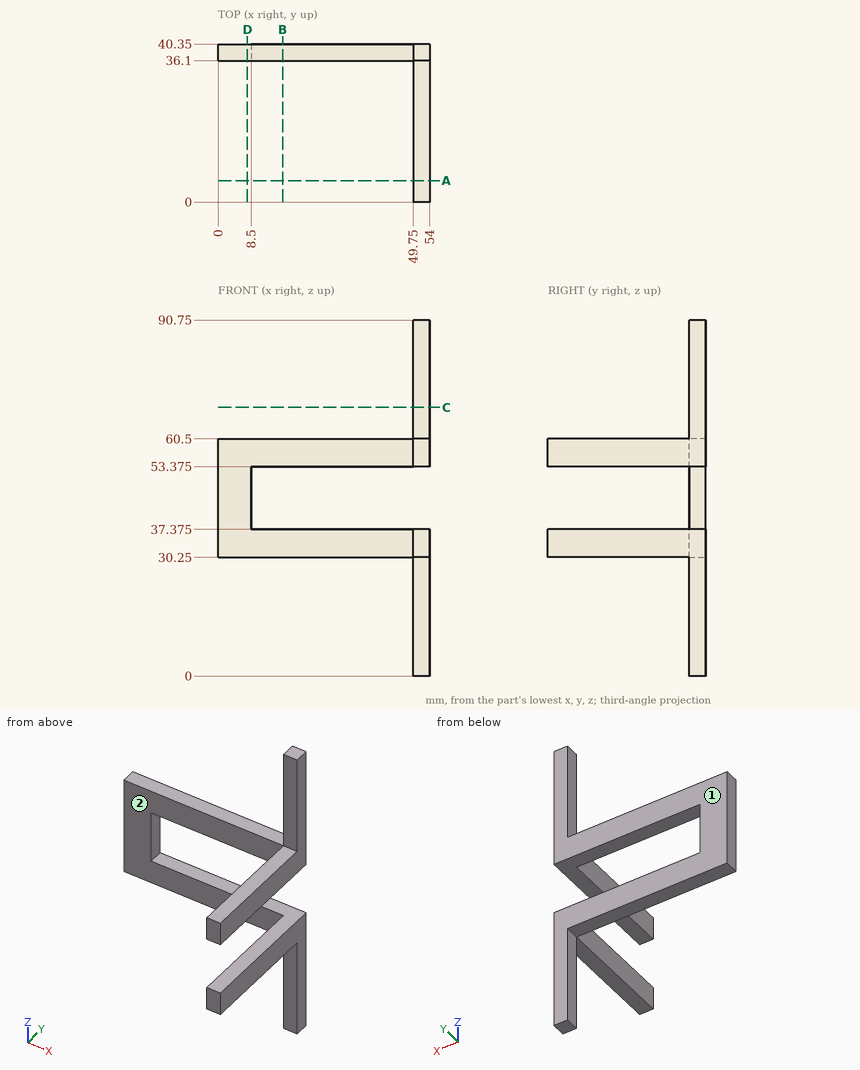
Source: three-view drawing plus pictorial views. Frame: mm from the lowest corner of the part. A direction names the side the tool comes from. Round coordinates to 2 decimals unless told otherwise and drop trailing zeros. Order: outer loops, then holes, each group sorted by start corner. A loop starts at its lowest first (then second) coordinate and runs counter-clockwise, first axis right, second up. Notation, with made-up numbers: (65, 15) -> (88, 15) arc R20 cw to (88, 40) -> close; hole circle Ø6 at (47.5, 0.5). An arc over 180 degrees is marked (long way). Use one line per item in the form item = value.
(1) Section C-C on z = 68.5. Return loops of the section in (x, y), and give its area (3 significant figures).
Results list:
outline = (49.75, 36.1) -> (54, 36.1) -> (54, 40.35) -> (49.75, 40.35) -> close
area = 18.1 mm^2
(2) Access query for the marked faces 1 and 2. Directions: +Z, -Z, +X, -X, +Y, -Y. A direction counts if a zero-diameter tool reaches every point of the face in a straight line with its end or side. Return the directions, or none.
Results list:
face_1 = +Z, -Z, +X, -X, +Y
face_2 = +Z, -Z, -X, -Y
(3) Section A-A on y = 5.5. Return loops of the section in (x, z) (3 decimals).
Results list:
outline = (49.75, 30.25) -> (54, 30.25) -> (54, 37.375) -> (49.75, 37.375) -> close; (49.75, 53.375) -> (54, 53.375) -> (54, 60.5) -> (49.75, 60.5) -> close
(4) First-contact query: pin 1 Ø1.3 at (x, z) = (51, 20) entering from -Y; pin 2 Ø8 at (y, z) = (21.5, 57) entering from -X; pin 3 Ø4.5 at (x, y) = (16.5, 39) entering from -Z. Flat tips, straight axial feed; report the tip coordinate or a pass-through.
Results list:
pin_1 = 36.1
pin_2 = 49.75
pin_3 = 30.25
(5) Section D-D on x = 7.5. Return loops of the section in (y, z), and give its area (3 significant figures).
Results list:
outline = (36.1, 30.25) -> (40.35, 30.25) -> (40.35, 60.5) -> (36.1, 60.5) -> close
area = 129 mm^2
(6) Section B-B on x = 16.5. Return loops of the section in (y, z) (3 decimals), and give its area (3 significant figures).
Results list:
outline = (36.1, 30.25) -> (40.35, 30.25) -> (40.35, 37.375) -> (36.1, 37.375) -> close; (36.1, 53.375) -> (40.35, 53.375) -> (40.35, 60.5) -> (36.1, 60.5) -> close
area = 60.6 mm^2
(7) Ray query, probe 1 along X at (y, z) = (38.5, 51.5); probe 2 along X at (y, z) = (3, 53.5); probe 3 along Y at (x, z) = (16.5, 34). Return the intervals inside material, ascending. Write a range as [from, to].
Results list:
probe_1 = [0, 8.5]
probe_2 = [49.75, 54]
probe_3 = [36.1, 40.35]
